Part model, mm, in its own coordinate system. Give positions to 0.01 mm unless a question says otherwise; leave off trailing zeros. Loops run counter-clockwise (first coordinate to the right, second up) from the corner with the lowest first, then second, coordinate; pieces in that order, holes last. Notation, with made-up numbers: (86.5, 27) -> (125.5, 27) arc R21 cw to (125.5, 35) -> close; hole circle Ø8 at (14.25, 24). An arc over 180 degrees is marked (long way). One line per question, with ' | ' between items.
```python
from build123d import *

# Parameters (mm, degrees)
SKETCH_1_W          = 270
SKETCH_1_H          = 5
EXTRUDE_1_DEPTH     = 95
SKETCH_2_R          = 2.25
SKETCH_2_R_2        = 17.5
CUT_EXTRUDE_1_DEPTH = 10
SKETCH_3_W          = 70
SKETCH_3_H          = 20
CUT_EXTRUDE_2_DEPTH = 10
FILLET_1_R          = 10
SKETCH_4_R          = 2.75
SKETCH_4_W          = 5
SKETCH_4_H          = 20
CUT_EXTRUDE_3_DEPTH = 10
SKETCH_5_R          = 1.55
CUT_EXTRUDE_4_DEPTH = 10


with BuildPart() as part:
    # 草图1 → 拉伸-薄壁1 (new body)
    with BuildSketch(Plane.XY):
        with Locations((-135, -2.5)):
            Rectangle(SKETCH_1_W, SKETCH_1_H)
    extrude(amount=EXTRUDE_1_DEPTH)

    # 草图2 → 切除-拉伸1 (cut)
    with BuildSketch(Plane(origin=(0, 0, 0), x_dir=(1, 0, 0), z_dir=(0, 1, 0))):
        with Locations(Location((-246, -25.75, 0), (0, 0, 270))):
            Circle(SKETCH_2_R)
        with Locations(Location((-229.338533362, -33.519369489, 0), (0, 0, 270))):
            Circle(SKETCH_2_R)
        with Locations(Location((-262.661466638, -33.519369489, 0), (0, 0, 270))):
            Circle(SKETCH_2_R)
        with Locations(Location((-262.661466638, -61.480630511, 0), (0, 0, 270))):
            Circle(SKETCH_2_R)
        with Locations(Location((-246, -69.25, 0), (0, 0, 270))):
            Circle(SKETCH_2_R)
        with Locations(Location((-229.338533362, -61.480630511, 0), (0, 0, 270))):
            Circle(SKETCH_2_R)
        with Locations(Location((-246, -47.5, 0), (0, 0, 270))):
            Circle(SKETCH_2_R_2)
    extrude(amount=-CUT_EXTRUDE_1_DEPTH, mode=Mode.SUBTRACT)

    # 草图3 → 切除-拉伸2 (cut)
    with BuildSketch(Plane(origin=(0, 0, 0), x_dir=(1, 0, 0), z_dir=(0, 1, 0))):
        with Locations((-235, -85)):
            Rectangle(SKETCH_3_W, SKETCH_3_H)
        with Locations((-235, -10)):
            Rectangle(SKETCH_3_W, SKETCH_3_H)
        with BuildLine():
            Line((-190, -10), (-190, -34.757359313))
            ThreePointArc((-190, -34.757359313), (-188.148050297, -37.52899791), (-184.878679656, -36.878679656))
            Line((-184.878679656, -36.878679656), (-160.121320344, -12.121320344))
            ThreePointArc((-160.121320344, -12.121320344), (-159.47100209, -8.851949703), (-162.242640687, -7))
            Line((-162.242640687, -7), (-187, -7))
            ThreePointArc((-187, -7), (-189.121320344, -7.878679656), (-190, -10))
        make_face()
        with BuildLine():
            Line((-154.121320344, -12.121320344), (-178.878679656, -36.878679656))
            ThreePointArc((-178.878679656, -36.878679656), (-179.52899791, -40.148050297), (-176.757359313, -42))
            Line((-176.757359313, -42), (-152, -42))
            ThreePointArc((-152, -42), (-149.878679656, -41.121320344), (-149, -39))
            Line((-149, -39), (-149, -14.242640687))
            ThreePointArc((-149, -14.242640687), (-150.851949703, -11.47100209), (-154.121320344, -12.121320344))
        make_face()
        with BuildLine():
            Line((-112.242640687, -7), (-137, -7))
            ThreePointArc((-137, -7), (-139.121320344, -7.878679656), (-140, -10))
            Line((-140, -10), (-140, -34.757359313))
            ThreePointArc((-140, -34.757359313), (-138.148050297, -37.52899791), (-134.878679656, -36.878679656))
            Line((-134.878679656, -36.878679656), (-110.121320344, -12.121320344))
            ThreePointArc((-110.121320344, -12.121320344), (-109.47100209, -8.851949703), (-112.242640687, -7))
        make_face()
        with BuildLine():
            Line((-99, -39), (-99, -14.242640687))
            ThreePointArc((-99, -14.242640687), (-100.851949703, -11.47100209), (-104.121320344, -12.121320344))
            Line((-104.121320344, -12.121320344), (-128.878679656, -36.878679656))
            ThreePointArc((-128.878679656, -36.878679656), (-129.52899791, -40.148050297), (-126.757359313, -42))
            Line((-126.757359313, -42), (-102, -42))
            ThreePointArc((-102, -42), (-99.878679656, -41.121320344), (-99, -39))
        make_face()
        with BuildLine():
            Line((-112.242640687, -52), (-137, -52))
            ThreePointArc((-137, -52), (-139.121320344, -52.878679656), (-140, -55))
            Line((-140, -55), (-140, -79.757359313))
            ThreePointArc((-140, -79.757359313), (-138.148050297, -82.52899791), (-134.878679656, -81.878679656))
            Line((-134.878679656, -81.878679656), (-110.121320344, -57.121320344))
            ThreePointArc((-110.121320344, -57.121320344), (-109.47100209, -53.851949703), (-112.242640687, -52))
        make_face()
        with BuildLine():
            Line((-99, -84), (-99, -59.242640687))
            ThreePointArc((-99, -59.242640687), (-100.851949703, -56.47100209), (-104.121320344, -57.121320344))
            Line((-104.121320344, -57.121320344), (-128.878679656, -81.878679656))
            ThreePointArc((-128.878679656, -81.878679656), (-129.52899791, -85.148050297), (-126.757359313, -87))
            Line((-126.757359313, -87), (-102, -87))
            ThreePointArc((-102, -87), (-99.878679656, -86.121320344), (-99, -84))
        make_face()
        with BuildLine():
            Line((-162.242640687, -52), (-187, -52))
            ThreePointArc((-187, -52), (-189.121320344, -52.878679656), (-190, -55))
            Line((-190, -55), (-190, -79.757359313))
            ThreePointArc((-190, -79.757359313), (-188.148050297, -82.52899791), (-184.878679656, -81.878679656))
            Line((-184.878679656, -81.878679656), (-160.121320344, -57.121320344))
            ThreePointArc((-160.121320344, -57.121320344), (-159.47100209, -53.851949703), (-162.242640687, -52))
        make_face()
        with BuildLine():
            Line((-149, -84), (-149, -59.242640687))
            ThreePointArc((-149, -59.242640687), (-150.851949703, -56.47100209), (-154.121320344, -57.121320344))
            Line((-154.121320344, -57.121320344), (-178.878679656, -81.878679656))
            ThreePointArc((-178.878679656, -81.878679656), (-179.52899791, -85.148050297), (-176.757359313, -87))
            Line((-176.757359313, -87), (-152, -87))
            ThreePointArc((-152, -87), (-149.878679656, -86.121320344), (-149, -84))
        make_face()
        with BuildLine():
            Line((-62.242640687, -7), (-87, -7))
            ThreePointArc((-87, -7), (-89.121320344, -7.878679656), (-90, -10))
            Line((-90, -10), (-90, -34.757359313))
            ThreePointArc((-90, -34.757359313), (-88.148050297, -37.52899791), (-84.878679656, -36.878679656))
            Line((-84.878679656, -36.878679656), (-60.121320344, -12.121320344))
            ThreePointArc((-60.121320344, -12.121320344), (-59.47100209, -8.851949703), (-62.242640687, -7))
        make_face()
        with BuildLine():
            Line((-49, -39), (-49, -14.242640687))
            ThreePointArc((-49, -14.242640687), (-50.851949703, -11.47100209), (-54.121320344, -12.121320344))
            Line((-54.121320344, -12.121320344), (-78.878679656, -36.878679656))
            ThreePointArc((-78.878679656, -36.878679656), (-79.52899791, -40.148050297), (-76.757359313, -42))
            Line((-76.757359313, -42), (-52, -42))
            ThreePointArc((-52, -42), (-49.878679656, -41.121320344), (-49, -39))
        make_face()
        with BuildLine():
            Line((-62.242640687, -52), (-87, -52))
            ThreePointArc((-87, -52), (-89.121320344, -52.878679656), (-90, -55))
            Line((-90, -55), (-90, -79.757359313))
            ThreePointArc((-90, -79.757359313), (-88.148050297, -82.52899791), (-84.878679656, -81.878679656))
            Line((-84.878679656, -81.878679656), (-60.121320344, -57.121320344))
            ThreePointArc((-60.121320344, -57.121320344), (-59.47100209, -53.851949703), (-62.242640687, -52))
        make_face()
        with BuildLine():
            Line((-49, -84), (-49, -59.242640687))
            ThreePointArc((-49, -59.242640687), (-50.851949703, -56.47100209), (-54.121320344, -57.121320344))
            Line((-54.121320344, -57.121320344), (-78.878679656, -81.878679656))
            ThreePointArc((-78.878679656, -81.878679656), (-79.52899791, -85.148050297), (-76.757359313, -87))
            Line((-76.757359313, -87), (-52, -87))
            ThreePointArc((-52, -87), (-49.878679656, -86.121320344), (-49, -84))
        make_face()
    extrude(amount=-CUT_EXTRUDE_2_DEPTH, mode=Mode.SUBTRACT)

    # 圆角1
    fillet_1_edges = [part.edges().sort_by_distance(p)[0] for p in [
        (-200, -2.5, 95),
        (-200, -2.5, 0),
        (-200, -2.5, 20),
        (-200, -2.5, 75),
        (-270, -2.5, 75),
        (-270, -2.5, 20),
    ]]
    fillet(fillet_1_edges, radius=FILLET_1_R - 0.0001)  # a hair under: the kernel refuses the full size

    # 草图4 → 切除-拉伸3 (cut)
    with BuildSketch(Plane(origin=(0, 0, 0), x_dir=(1, 0, 0), z_dir=(0, 1, 0))):
        with Locations(Location((-20, -17.5, 0), (0, 0, 270))):
            Circle(SKETCH_4_R)
        with Locations(Location((-20, -47.5, 0), (0, 0, 270))):
            Circle(SKETCH_4_R)
        with Locations(Location((-20, -77.5, 0), (0, 0, 270))):
            Circle(SKETCH_4_R)
        with Locations((-2.5, -67.5)):
            Rectangle(SKETCH_4_W, SKETCH_4_H)
        with Locations((-2.5, -27.5)):
            Rectangle(SKETCH_4_W, SKETCH_4_H)
    extrude(amount=-CUT_EXTRUDE_3_DEPTH, mode=Mode.SUBTRACT)

    # 草图5 → 切除-拉伸4 (cut)
    with BuildSketch(Plane(origin=(0, 0, 0), x_dir=(1, 0, 0), z_dir=(0, 1, 0))):
        with Locations((-5, -19.05)):
            Circle(SKETCH_5_R)
        with Locations((-5, -35.95)):
            Circle(SKETCH_5_R)
        with Locations((-5, -59.05)):
            Circle(SKETCH_5_R)
        with Locations((-5, -75.95)):
            Circle(SKETCH_5_R)
    extrude(amount=-CUT_EXTRUDE_4_DEPTH, mode=Mode.SUBTRACT)


solid = part.part
```
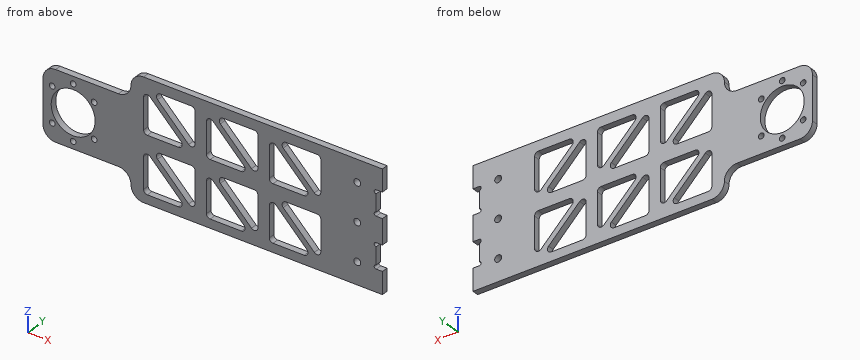
1) Saw through at D-D (y = -2.1). State how many separate pieces and enclosed holes the cut face has, and give its area (3 significant figures).
Found:
separate pieces: 1 | enclosed holes: 22 | area: 14,400 mm2
2) Pin check, flat tips, straight feed: P1, Ø2.5, axis at y = -3, z = 21, coming from the -X side; P2, Ø1.5, axis at y = -2, z = 27.5, coming from the +X side; P3, Ø1.5, axis at y = -2.5, z = 74, coming from the -X side. Stop position of each tip, or through.
Found:
P1: x = -266.32 | P2: x = -5 | P3: x = -265.65
3) Drill centre lines: line 1 (Z direction, x = -124, y = -4.65); line 2 (X direction, y = -2.15, z = 41); line 3 (Z direction, x = -129.5, y = -3.8). Where is each one in solid material? Low to high.
Found:
line 1: 0 to 7, 26 to 32, 42 to 52, 71 to 77, 87 to 95 | line 2: -270 to -262.25, -229.75 to -178.99, -149.76 to -128.99, -99.76 to -78.99, -49.76 to 0 | line 3: 0 to 7, 31.5 to 37.78, 40.22 to 52, 76.5 to 82.78, 85.22 to 95
4) Saw through at A-A (x = -124). Give the cut face in (y, z).
Found:
outline: (-5, 0) -> (0, 0) -> (0, 7) -> (-5, 7) -> close; (-5, 26) -> (0, 26) -> (0, 32) -> (-5, 32) -> close; (-5, 42) -> (0, 42) -> (0, 52) -> (-5, 52) -> close; (-5, 71) -> (0, 71) -> (0, 77) -> (-5, 77) -> close; (-5, 87) -> (0, 87) -> (0, 95) -> (-5, 95) -> close
5) Saw through at B-B (z = 47.5). Give the cut face in (x, y).
Found:
outline: (-270, -5) -> (-263.5, -5) -> (-263.5, 0) -> (-270, 0) -> close; (-228.5, -5) -> (-22.75, -5) -> (-22.75, 0) -> (-228.5, 0) -> close; (-17.25, -5) -> (0, -5) -> (0, 0) -> (-17.25, 0) -> close
6) Saw through at C-C (x = -216.5). Give the cut face in (y, z).
Found:
outline: (-5, 20) -> (0, 20) -> (0, 75) -> (-5, 75) -> close
